from build123d import *

# Parameters (mm, degrees)
SKETCH1_W           = 36
SKETCH1_H           = 12
SKETCH1_R           = 4
BOSS_EXTRUDE1_DEPTH = 5
SKETCH2_W           = 36
SKETCH2_H           = 12
BOSS_EXTRUDE2_DEPTH = 3
CHAMFER3_SIZE       = 3


with BuildPart() as part:
    # Sketch1 → Boss-Extrude1 (new body)
    with BuildSketch(Plane(origin=(0, 0, 0), x_dir=(1, 0, 0), z_dir=(0, 1, 0))):
        Rectangle(SKETCH1_W, SKETCH1_H)
        with Locations(Location((11.845, 0, 0), (0, 0, 270))):
            Circle(SKETCH1_R, mode=Mode.SUBTRACT)
        with Locations(Location((-11.845, 0, 0), (0, 0, 270))):
            Circle(SKETCH1_R, mode=Mode.SUBTRACT)
    extrude(amount=-BOSS_EXTRUDE1_DEPTH)

    # Sketch2 → Boss-Extrude2 (add)
    with BuildSketch(Plane(origin=(0, 0, 0), x_dir=(1, 0, 0), z_dir=(0, 1, 0))):
        Rectangle(SKETCH2_W, SKETCH2_H)
    extrude(amount=BOSS_EXTRUDE2_DEPTH)

    # Chamfer3
    chamfer3_edges = [part.edges().sort_by_distance(p)[0] for p in [
        (18, -1, 6),
        (-18, -1, 6),
        (-18, -1, -6),
        (18, -1, -6),
    ]]
    chamfer(chamfer3_edges, length=CHAMFER3_SIZE)


solid = part.part
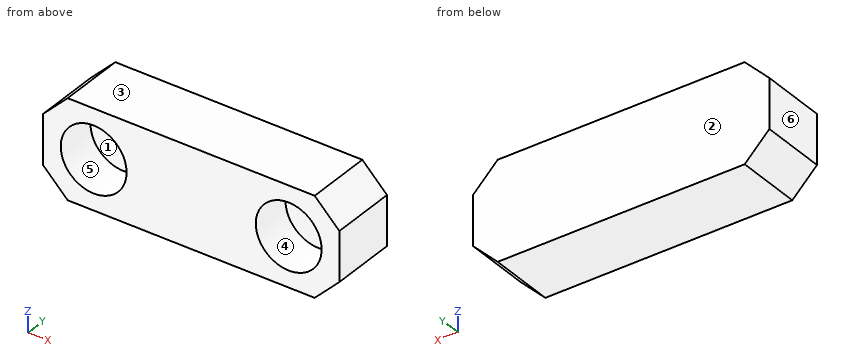
Verification items for the finished model (mm, model axes). Face numbers are marked on the shaded views. A direction names the side the tool comes from. Give positions to 0.01 mm unless a question says otherwise; leave off trailing zeros. Loops run counter-clockwise (first coordinate to the right, second up) from the corner with the lowest first, then second, coordinate; pieces in that order, holes last.
1. Material ranges on probe 1 along X at (y, z) = (-3.4, 0) (3 decimals); probe 2 along X at (y, z) = (-1.5, -2.5); probe 3 along Z at (x, y) = (-12, -0.5), recorded low to high.
Derived:
probe 1: x = -18 to -15.845, -7.845 to 7.845, 15.845 to 18
probe 2: x = -18 to -14.97, -8.72 to 8.72, 14.97 to 18
probe 3: z = -6 to -4, 4 to 6
2. Tool access check on the marked faces 1 and 2. Record the directions out of +Z, -Z, +X, -X, +Y, -Y that give a thin tool (end or side, any length) a straight path to the whole face; none if there is none.
Derived:
face 1: -Y
face 2: +Z, -Z, +X, -X, +Y
3. Release check for a two-part mould opening along Z. For the marked faces 3, 4, 5 and 6 record: +Z half, -Z half, draft (parallel to the pull), parting line (faces both ways), or undercut.
Derived:
face 3: +Z half
face 4: undercut
face 5: undercut
face 6: draft
4. Cross-section at B-B on z = 0. Record the cut outline in (x, y) (3 decimals), and give its area (3 significant figures).
Derived:
outline: (-18, -5) - (-15.845, -5) - (-15.845, 0) - (-7.845, 0) - (-7.845, -5) - (7.845, -5) - (7.845, 0) - (15.845, 0) - (15.845, -5) - (18, -5) - (18, 3) - (-18, 3) - close
area: 208 mm2
5. Cross-section at D-D on y = -3.5. Record the cut outline in (x, z) (3 decimals).
Derived:
outline: (-18, -3) - (-15, -6) - (15, -6) - (18, -3) - (18, 3) - (15, 6) - (-15, 6) - (-18, 3) - close; hole circle Ø8 at (-11.845, 0); hole circle Ø8 at (11.845, 0)
6. Cross-section at C-C on x = 13. Record the cut outline in (y, z), and give its area (3 significant figures).
Derived:
outline: (-5, -6) - (3, -6) - (3, 6) - (-5, 6) - (-5, 3.83) - (0, 3.83) - (0, -3.83) - (-5, -3.83) - close
area: 57.7 mm2
7. Go/stop test with a flat-tipped pin: P1, Ø1, axis at x = -12.5, z = 0.5, coming from the -Y side. Record where the tip stops, or that it passes through.
Derived:
P1: stops at y = 0
8. Cross-section at A-A on y = 1. Record the cut outline in (x, z).
Derived:
outline: (-18, -3) - (-15, -6) - (15, -6) - (18, -3) - (18, 3) - (15, 6) - (-15, 6) - (-18, 3) - close
